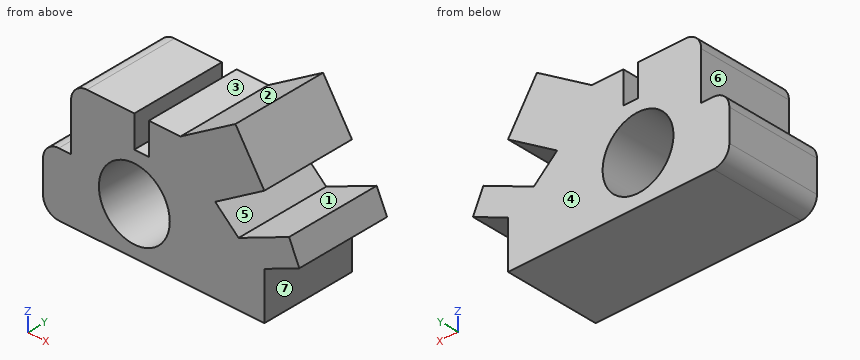
from build123d import *

# Parameters (mm, degrees)
F0_R     = 11.20644
F1_DEPTH = 30


with BuildPart() as f1:
    # F0 (on Front) → F1 (new body)
    with BuildSketch(Plane.XZ):
        with BuildLine():
            Line((-46.625002, -15), (18.374998, -15))
            Line((18.374998, -15), (18.374998, 0))
            Line((18.374998, 0), (29.448327, 5))
            Line((29.448327, 5), (26.193243, 12.208923))
            Line((26.193243, 12.208923), (10.227887, 5))
            Line((10.227887, 5), (2.843751, 11.743481))
            Line((2.843751, 11.743481), (18.374998, 21.587231))
            Line((18.374998, 21.587231), (9.231542, 36.01357))
            Line((9.231542, 36.01357), (-8.145421, 25))
            Line((-8.145421, 25), (-18.145421, 25))
            Line((-18.145421, 25), (-18.145421, 15))
            Line((-18.145421, 15), (-22.739174, 15))
            Line((-22.739174, 15), (-22.739174, 25))
            Line((-22.739174, 25), (-37.739174, 25))
            ThreePointArc((-37.739174, 25), (-41.274708, 23.535534), (-42.739174, 20))
            Line((-42.739174, 20), (-42.739174, 5))
            Line((-42.739174, 5), (-46.625002, 5))
            ThreePointArc((-46.625002, 5), (-50.160536, 3.535534), (-51.625002, 0))
            Line((-51.625002, 0), (-51.625002, -10))
            ThreePointArc((-51.625002, -10), (-50.160536, -13.535534), (-46.625002, -15))
        make_face()
        with Locations((-22.739174, 0)):
            Circle(F0_R, mode=Mode.SUBTRACT)
    extrude(amount=F1_DEPTH)


solid = f1.part
Check sheet for the modelled part. Datum: model origin and axes. Units: mm. Face numbers are marked on the shaded views. A direction names the side the tool comes from. Coordinates: 2 decimals unless noted, no trailing zeros. Write each loop counter-clockwise with the first axis right and the second up, starting at its lowest first coordinate (ties: lowest second). Pieces come first, ordered by that corner, then holes.
Item 1: Depth check by flat-ended pin: pin 1 Ø8 at (x, y) = (-13, -14.5) entering from +Z; pin 2 Ø8 at (x, y) = (3.5, -14) entering from +Z; pin 3 Ø16.5 at (y, z) = (-9, -4) entering from +X. Enter the tip coordinate at first touch or a pass-through.
Numbers:
pin 1: stops at z = 25
pin 2: stops at z = 34.92
pin 3: stops at x = 27.79
Item 2: Scan lines: probe 1 along X at (y, z) = (-8, 10); probe 2 along Z at (x, y) = (-8.5, -9); probe 3 along X at (y, z) = (-6.5, -6) (3 decimals). Record each from-to range of solid material in increasing order.
Numbers:
probe 1: x = -42.74 to -27.8, -17.68 to 4.75, 21.3 to 27.19
probe 2: z = -15 to 25
probe 3: x = -51.625 to -32.204, -13.274 to 18.375
Item 3: Cross-section at A-A on y = -15. Record the boundary of the cut face in (x, z) (3 decimals), then the cut area to 3 significant figures.
Numbers:
outline: (-51.625, -10) arc R5 ccw to (-46.625, -15) - (18.375, -15) - (18.375, 0) - (29.448, 5) - (26.193, 12.209) - (10.228, 5) - (2.844, 11.743) - (18.375, 21.587) - (9.232, 36.014) - (-8.145, 25) - (-18.145, 25) - (-18.145, 15) - (-22.739, 15) - (-22.739, 25) - (-37.739, 25) arc R5 ccw to (-42.739, 20) - (-42.739, 5) - (-46.625, 5) arc R5 ccw to (-51.625, 0) - close; hole circle Ø22.413 at (-22.739, 0)
area: 2,240 mm2
Item 4: Access from +Z, -Z, +X, -X, +Y, -Y to the whole of each face (thin tool, end or side, straight path). Record for the marked faces 4, 5, 6 and 7.
Numbers:
face 4: +Z, -Z, +X, -X, +Y
face 5: +Y, -Y
face 6: +Z, -X, +Y, -Y
face 7: -Z, +X, +Y, -Y
Item 5: Cross-section at D-D on x = -45. Record the boundary of the cut face in (y, z), then the cut area to 3 significant figures.
Numbers:
outline: (-30, -15) - (0, -15) - (0, 5) - (-30, 5) - close
area: 600 mm2
Item 6: Cross-section at C-C on x = -27. Record the boundary of the cut face in (y, z), then the cut area to 3 significant figures.
Numbers:
outline: (-30, -15) - (0, -15) - (0, -10.36) - (-30, -10.36) - close; (-30, 10.36) - (0, 10.36) - (0, 25) - (-30, 25) - close
area: 578 mm2
Item 7: Cross-section at B-B on z = 1. Record the boundary of the cut face in (x, y), then the cut area to 3 significant figures.
Numbers:
outline: (-51.52, -30) - (-33.9, -30) - (-33.9, 0) - (-51.52, 0) - close; (-11.58, -30) - (20.59, -30) - (20.59, 0) - (-11.58, 0) - close
area: 1,490 mm2
Item 8: Mould release check, pull along X, two halves, no side actions. Record for the marked faces 1, 2 and 3: released by +X, released by -X, zero draft, split by the parting line, or undercut.
Numbers:
face 1: undercut
face 2: released by -X
face 3: zero draft
